Source: three-view drawing plus pictorial views. Frame: mm from the lowest corner of the part. A direction names the side the tool comes from. Give positions to 0.01 mm unless a question says otherwise; leave off trailing zeros. Order: outer loops, then holes, each group sorted by start corner. A loop starts at its lowest first (then second) coordinate and runs counter-clockwise, first axis right, second up. Notation, with made-up numbers: (58, 43.25) -> (96, 43.25) arc R7 ccw to (96, 47.25) -> close; hole circle Ø7 at (80.5, -37). An arc over 180 degrees is marked (long way). One line per question, with ' | ' between items.
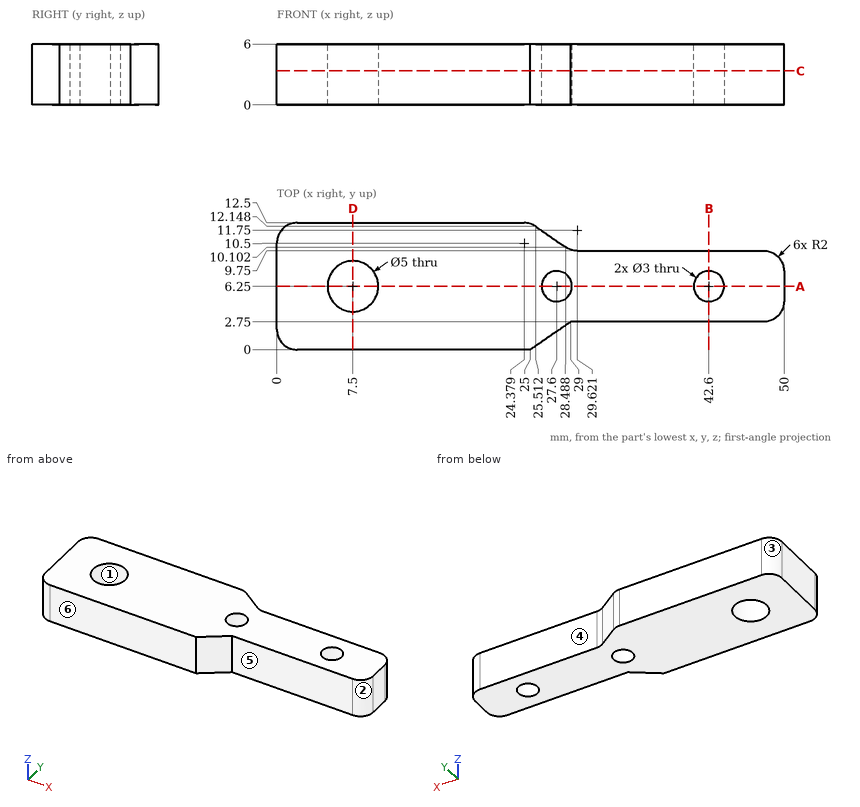
1) Section A-A on y = 6.25. Return loops of the section in (x, z).
Check result:
outline: (0, 0) -> (5, 0) -> (5, 6) -> (0, 6) -> close; (10, 0) -> (26.1, 0) -> (26.1, 6) -> (10, 6) -> close; (29.1, 0) -> (41.1, 0) -> (41.1, 6) -> (29.1, 6) -> close; (44.1, 0) -> (50, 0) -> (50, 6) -> (44.1, 6) -> close
2) Section D-D on x = 7.5. Return loops of the section in (y, z), plus the area to 3 significant figures.
Check result:
outline: (0, 0) -> (3.75, 0) -> (3.75, 6) -> (0, 6) -> close; (8.75, 0) -> (12.5, 0) -> (12.5, 6) -> (8.75, 6) -> close | area: 45.0 mm^2
3) Set-up query: the marked faces 4, 5 and 6. Return all of +Z, -Z, +X, -X, +Y, -Y with unobstructed straight access to the full face (end or side cutting, diameter ignored); none if empty.
Check result:
face 4: +Z, -Z, +X, +Y | face 5: +Z, -Z, +X, -Y | face 6: +Z, -Z, +X, -X, -Y
4) Section C-C on z = 3.35. Return loops of the section in (x, y).
Check result:
outline: (0, 2) arc R2 ccw to (2, 0) -> (25, 0) -> (29, 2.75) -> (48, 2.75) arc R2 ccw to (50, 4.75) -> (50, 7.75) arc R2 ccw to (48, 9.75) -> (29.62, 9.75) arc R2 cw to (28.49, 10.1) -> (25.51, 12.15) arc R2 ccw to (24.38, 12.5) -> (2, 12.5) arc R2 ccw to (0, 10.5) -> close; hole circle Ø5 at (7.5, 6.25); hole circle Ø3 at (27.6, 6.25); hole circle Ø3 at (42.6, 6.25)
5) Section B-B on x = 42.6. Return loops of the section in (y, z).
Check result:
outline: (2.75, 0) -> (4.75, 0) -> (4.75, 6) -> (2.75, 6) -> close; (7.75, 0) -> (9.75, 0) -> (9.75, 6) -> (7.75, 6) -> close
6) Material intervals for probe 1 along Y at (x, z) = (5.5, 4.25); probe 2 along Y at (x, z) = (7.5, 3.5); probe 3 along X at (y, z) = (5.25, 0.5), sorted ascending. Write a range as from..to.
Check result:
probe 1: y = 0..4.75, 7.75..12.5 | probe 2: y = 0..3.75, 8.75..12.5 | probe 3: x = 0..5.21, 9.79..26.48, 28.72..41.48, 43.72..50
7) Contact query for a flat-ended pin moving along its axis: pin 1 Ø1.8 at (x, z) = (37.5, 3) entering from -Y. Output: stop coordinate, or through.
Check result:
pin 1: stops at y = 2.75
8) Pull-direction query (Y, two-part tool) for the marked faces 1, 2 and 3; classes: +Y half, -Y half, draft (parallel to the pull), parting line (faces both ways), or undercut.
Check result:
face 1: undercut | face 2: -Y half | face 3: +Y half
